Read the model definition and answer for the solid it produces. Units are mm, in the model's axes. Face numbers are marked on the shaded views. A direction names the side the tool comes from. Coordinates: 2 decimals unless noted, no trailing zeros. Write each loop counter-clockwise with the first axis right and the second up, starting at its lowest first coordinate (ties: lowest second). Pieces come first, ordered by that corner, then holes. Notation, with made-up numbers: (6.25, 27) -> (16.25, 27) arc R34 cw to (16.25, 62) -> close; hole circle Ø4 at (51, 11). An arc over 180 degrees is marked (long way). Write item = value, one per line. Start each with the question number.
1) A tool of negligible diameter and unlimited length cuts with its end or side. For the marked faces 1 and 2, from which of +Z, -Z, +X, -X, +Y, -Y can it reach the whole face along a straight path? Write none if from no direction.
2) Find the intervals of material crossed by line 1 along Y through (x, z) = (-2, 2); line 2 along Z through (x, y) = (10.5, 11.5); line 3 along X through (y, z) = (1.5, 3.8), in increasing order. Write a range as from..to.
3) Flat-ended cylindrical pins translate along their axes: pin 1 Ø10 at (x, y) = (-13.5, 3.5) entering from +Z; pin 2 Ø1.2 at (x, z) = (15.5, 1.5) entering from -Y; pin 3 Ø2 at (x, z) = (7.5, 1) entering from +Y. Find the tip coordinate at first contact, or state that the pin passes through.
4) Section B-B (x = 0) is taken. Determine the outline of the cut face in (y, z).
5) Section A-A (z = 1.55) is taken. Determine the outline of the cut face in (x, y), plus the area to 3 significant figures.
from build123d import *

# Parameters (mm, degrees)
CROQUIS1_W              = 64
CROQUIS1_H              = 33
SALIENTE_EXTRUIR1_DEPTH = 2.5
CROQUIS3_W              = 5
CROQUIS3_H              = 37
SALIENTE_EXTRUIR2_DEPTH = 3.5
REDONDEO1_R             = 2
CROQUIS4_W              = 0.2
CROQUIS4_H              = 37
CORTAR_EXTRUIR1_DEPTH   = 0.5
REDONDEO2_R             = 0.1


with BuildPart() as part:
    # Croquis1 → Saliente-Extruir1 (new body)
    with BuildSketch(Plane.XY):
        Rectangle(CROQUIS1_W, CROQUIS1_H)
    extrude(amount=SALIENTE_EXTRUIR1_DEPTH)

    # Croquis3 → Saliente-Extruir2 (add)
    with BuildSketch(Plane.ZY.offset(32)):
        with Locations((2.5, 0)):
            Rectangle(CROQUIS3_W, CROQUIS3_H)
    extrude(amount=SALIENTE_EXTRUIR2_DEPTH)

    # Redondeo1
    redondeo1_edges = [part.edges().sort_by_distance(p)[0] for p in [
        (-35.5, 18.5, 2.5),
        (-35.5, -18.5, 2.5),
    ]]
    fillet(redondeo1_edges, radius=REDONDEO1_R)

    # Croquis4 → Cortar-Extruir1 (cut)
    with BuildSketch(Plane.XY.offset(5)):
        with Locations((-32.3, 0)):
            Rectangle(CROQUIS4_W, CROQUIS4_H)
        with Locations((-32.8, 0)):
            Rectangle(CROQUIS4_W, CROQUIS4_H)
        with Locations((-33.3, 0)):
            Rectangle(CROQUIS4_W, CROQUIS4_H)
        with Locations((-33.8, 0)):
            Rectangle(CROQUIS4_W, CROQUIS4_H)
        with Locations((-34.3, 0)):
            Rectangle(CROQUIS4_W, CROQUIS4_H)
        with Locations((-34.8, 0)):
            Rectangle(CROQUIS4_W, CROQUIS4_H)
        with Locations((-35.3, 0)):
            Rectangle(CROQUIS4_W, CROQUIS4_H)
    extrude(amount=-CORTAR_EXTRUIR1_DEPTH, mode=Mode.SUBTRACT)

    # Redondeo2
    redondeo2_edges = [part.edges().sort_by_distance(p)[0] for p in [
        (-34.2, 0, 5),
        (-34.4, 0, 5),
        (-34.7, 0, 5),
        (-34.9, 0, 5),
        (-35.2, 0, 5),
        (-32, 0, 5),
        (-33.45, 18.5, 5),
        (-33.45, -18.5, 5),
        (-33.60012555, 18.497492146, 5),
        (-34.051681951, 18.422406571, 5),
        (-34.554113045, 18.199660463, 5),
        (-35.061282751, 17.749958468, 5),
        (-35.061282751, -17.749958468, 5),
        (-34.554113045, -18.199660463, 5),
        (-34.051681951, -18.422406571, 5),
        (-33.60012555, -18.497492146, 5),
        (-33.05, -18.5, 5),
        (-32.55, -18.5, 5),
        (-32.1, -18.5, 5),
        (-33.05, 18.5, 5),
        (-32.55, 18.5, 5),
        (-32.1, 18.5, 5),
        (-32.4, 0, 5),
        (-32.2, 0, 5),
        (-32.9, 0, 5),
        (-32.7, 0, 5),
        (-33.4, 0, 5),
        (-33.2, 0, 5),
        (-33.7, 0, 5),
        (-33.9, 0, 5),
    ]]
    fillet(redondeo2_edges, radius=REDONDEO2_R - 0.0001)  # a hair under: the kernel refuses the full size


solid = part.part
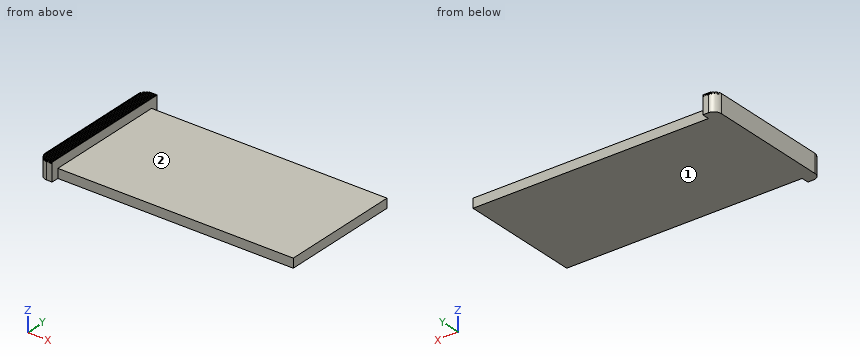
Answer key:
q1.face_1 = -Z, +X, -X, +Y, -Y
q1.face_2 = +Z, +X, +Y, -Y
q2.line_1 = -16.5..16.5
q2.line_2 = 0..2.5
q2.line_3 = -35.5..-32
q3.pin_1 = 2.5
q3.pin_2 = -16.5
q3.pin_3 = 16.5
q4.outline = (-16.5, 0) -> (16.5, 0) -> (16.5, 2.5) -> (-16.5, 2.5) -> close
q5.outline = (-35.5, -16.5) arc R2 ccw to (-33.5, -18.5) -> (-32, -18.5) -> (-32, -16.5) -> (32, -16.5) -> (32, 16.5) -> (-32, 16.5) -> (-32, 18.5) -> (-33.5, 18.5) arc R2 ccw to (-35.5, 16.5) -> close
q5.area = 2,240 mm^2
